```python
from build123d import *

# Parameters (mm, degrees)
CROQUIS1_W              = 28
CROQUIS1_H              = 12
SALIENTE_EXTRUIR1_DEPTH = 3
CROQUIS2_R              = 1
CORTAR_EXTRUIR1_DEPTH   = 3
CROQUIS3_W              = 3
CROQUIS3_H              = 8.392153605
SALIENTE_EXTRUIR2_DEPTH = 8
CROQUIS4_R              = 1
CORTAR_EXTRUIR2_DEPTH   = 3
CORTAR_EXTRUIR3_DEPTH   = 8
SALIENTE_EXTRUIR4_START = 0.5
CROQUIS11_R             = 1
SALIENTE_EXTRUIR4_DEPTH = 0.5
CROQUIS12_R             = 1
SALIENTE_EXTRUIR5_DEPTH = 0.5


with BuildPart() as part:
    # Croquis1 → Saliente-Extruir1 (new body)
    with BuildSketch(Plane.XY):
        with Locations((-16.412225504, 7.356643357)):
            Rectangle(CROQUIS1_W, CROQUIS1_H)
    extrude(amount=SALIENTE_EXTRUIR1_DEPTH)

    # Croquis2 → Cortar-Extruir1 (cut)
    with BuildSketch(Plane.XY.offset(3)):
        with Locations((-26.412225504, 5.356643357)):
            Circle(CROQUIS2_R)
        with Locations((-6.412225504, 5.356643357)):
            Circle(CROQUIS2_R)
    extrude(amount=-CORTAR_EXTRUIR1_DEPTH, mode=Mode.SUBTRACT)

    # Croquis3 → Saliente-Extruir2 (add)
    with BuildSketch(Plane(origin=(0, 0, 0), x_dir=(-1, 0, 0), z_dir=(0, 0, -1))):
        with Locations((16.412225504, 9.160566555)):
            Rectangle(CROQUIS3_W, CROQUIS3_H)
    extrude(amount=SALIENTE_EXTRUIR2_DEPTH)

    # Croquis4 → Cortar-Extruir2 (cut)
    with BuildSketch(Plane.ZY.offset(17.912225504)):
        with Locations((-4.5, 9.856643357)):
            Circle(CROQUIS4_R)
    extrude(amount=-CORTAR_EXTRUIR2_DEPTH, mode=Mode.SUBTRACT)

    # Croquis6 → Cortar-Extruir3 (cut)
    with BuildSketch(Plane.ZY.offset(17.912225504)):
        with BuildLine():
            Line((-8, 13.356643357), (-4.5, 13.356643357))
            Line((-4.5, 13.356643357), (0, 13.356643357))
            Line((0, 13.356643357), (0, 13.306643357))
            Line((0, 13.306643357), (-4.5, 13.306643357))
            ThreePointArc((-4.5, 13.306643357), (-7.95, 9.856643357), (-4.5, 6.406643357))
            Line((-4.5, 6.406643357), (0, 6.406643357))
            Line((0, 6.406643357), (0, 4.964489752))
            Line((0, 4.964489752), (-8, 4.964489752))
            Line((-8, 4.964489752), (-8, 6.352103478))
            Line((-8, 6.352103478), (-8, 13.356643357))
        make_face()
    extrude(amount=-CORTAR_EXTRUIR3_DEPTH, mode=Mode.SUBTRACT)

    # Croquis11 → Saliente-Extruir4 (add)
    with BuildSketch(Plane.ZY.offset(17.912225504).offset(SALIENTE_EXTRUIR4_START)):
        with BuildLine():
            Line((-4.5, 6.406643357), (0, 6.406643357))
            Line((0, 6.406643357), (0, 13.306643357))
            Line((0, 13.306643357), (-4.5, 13.306643357))
            ThreePointArc((-4.5, 13.306643357), (-7.95, 9.856643357), (-4.5, 6.406643357))
        make_face()
        with Locations((-4.5, 9.856643357)):
            Circle(CROQUIS11_R, mode=Mode.SUBTRACT)
    extrude(amount=-SALIENTE_EXTRUIR4_DEPTH)

    # Croquis12 → Saliente-Extruir5 (add)
    with BuildSketch(Plane(origin=(-14.912225504, 0, 0), x_dir=(0, 0, -1), z_dir=(1, 0, 0))):
        with BuildLine():
            Line((4.5, 13.306643357), (0, 13.306643357))
            Line((0, 13.306643357), (0, 6.406643357))
            Line((0, 6.406643357), (4.5, 6.406643357))
            ThreePointArc((4.5, 6.406643357), (7.95, 9.856643357), (4.5, 13.306643357))
        make_face()
        with Locations(Location((4.5, 9.856643357, 0), (0, 0, 180))):
            Circle(CROQUIS12_R, mode=Mode.SUBTRACT)
    extrude(amount=SALIENTE_EXTRUIR5_DEPTH)


solid = part.part
```
The listing builds one solid part. Answer for the finished solid, in the listing's coordinates (mm). A direction names the side the tool comes from. Give positions to 0.01 mm unless a question says otherwise; leave off trailing zeros. Order: outer loops, then holes, each group sorted by start corner. A loop starts at its lowest first (then second) coordinate and runs counter-clockwise, first axis right, second up. Notation, with made-up numbers: (65, -6.5) -> (86, -6.5) arc R32 cw to (86, 26.5) -> close; hole circle Ø11 at (77, -6.5). An arc over 180 degrees is marked (long way). Answer as a JSON object with one key per item and string values. Group by question number.
Item 1: A tool of negligible diameter and unlimited length cuts with its end or side. For faces 5 (the flat face through (-16, 13.307, -2)), 6 (the flat face through (-16, 6.407, -2)), 7 (the flat face through (-14.412, 10, -3)), from which of +Z, -Z, +X, -X, +Y, -Y can it reach the whole face along a straight path? Write none if from no direction.
Item 2: The part is cut by section A-A on y = 9.5. Write down the section's boundary in (x, z).
Item 3: Consider L1, parallel to X at y = 5.5, z = 1.75; L2, parallel to Z at x = -23.5, y = 3; L3, parallel to X at y = 9, z = -1.5. Determine where each line is inside the solid, lowest interval first. Write a range as from..to.
Item 4: The part is cut by section C-C on z = -4. Write down the section's boundary in (x, y), and give its area (3 significant figures).
Item 5: Flat-ended cylindrical pins translate along their axes: pin 1 (5.5 mm diameter, centred on y = 8, z = -3, fed in from +X); pin 2 (1.2 mm diameter, centred on x = -16.5, z = -1, fed in from +Y); pin 3 (6 mm diameter, centred on x = -26.5, y = 5, fed in from -Z); pin 4 (1.6 mm diameter, centred on y = 9.86, z = -4.5, fed in from +X). Find the tip coordinate at first contact, or state that the pin passes through.
Item 6: The part is cut by section D-D on y = 12.75. Write down the section's boundary in (x, z).
Item 7: Determine the mould class of faces 1 (the cylindrical face through (-7.41, 5.4, 1.52)), 2 (the cylindrical face through (-16.44, 9.78, -7.95)), 3 (the cylindrical face through (-16.44, 10.47, -5.29)), 4 (the flat face through (-17, 7, 3)) for opening direction Z: pulls with the +Z half, pulls with the -Z half, needs draft (parallel to the pull), parting line crosses it, or undercut.
Item 8: The part is cut by section B-B on x = -17.5. Write down the section's boundary in (y, z).
Result set:
{
 "1": {"face 5": "-Z, +X, -X, +Y", "face 6": "-Z, +X, -X, -Y", "face 7": "-Z, +X, +Y, -Y"},
 "2": {"outline": "(-30.41, 0) -> (-18.41, 0) -> (-18.41, -3.57) -> (-14.41, -3.57) -> (-14.41, 0) -> (-2.41, 0) -> (-2.41, 3) -> (-30.41, 3) -> close; (-18.41, -7.93) -> (-14.41, -7.93) -> (-14.41, -5.43) -> (-18.41, -5.43) -> close"},
 "3": {"L1": "-30.41..-27.4, -25.42..-7.4, -5.42..-2.41", "L2": "0..3", "L3": "-18.41..-14.41"},
 "4": {"outline": "(-18.41, 6.41) -> (-14.41, 6.41) -> (-14.41, 8.99) -> (-18.41, 8.99) -> close; (-18.41, 10.72) -> (-14.41, 10.72) -> (-14.41, 13.31) -> (-18.41, 13.31) -> close", "area": "20.7 mm²"},
 "5": {"pin 1": "x = -14.41", "pin 2": "y = 13.31", "pin 3": "z = 0", "pin 4": "through"},
 "6": {"outline": "(-30.41, 0) -> (-18.41, 0) -> (-18.41, -6.38) -> (-14.41, -6.38) -> (-14.41, 0) -> (-2.41, 0) -> (-2.41, 3) -> (-30.41, 3) -> close"},
 "7": {"face 1": "needs draft", "face 2": "pulls with the -Z half", "face 3": "undercut", "face 4": "pulls with the +Z half"},
 "8": {"outline": "(1.36, 0) -> (6.41, 0) -> (6.41, -4.5) arc R3.45 ccw to (13.31, -4.5) -> (13.31, 0) -> (13.36, 0) -> (13.36, 3) -> (1.36, 3) -> close; hole circle Ø2 at (9.86, -4.5)"}
}
